```python
from build123d import *

# Parameters (mm, degrees)
F1_DEPTH = 40.64
F2_W     = 58.1915168336
F2_H     = 84.6826420166
F3_DEPTH = 100.584
F4_DEPTH = 25.4
F5_R     = 11.938
F6_DEPTH = 25.4
F7_R     = 11.938
F8_DEPTH = 25.4


# Not quite as in the source:
# - a feature names something its author has since deleted; it is built from what else it names


with BuildPart() as f1:
    # F0 (on Front) → F1 (new body)
    with BuildSketch(Plane.XZ):
        Polygon((5.0445693985, -63.1324924332), (45.3936140645, -28.3097998209), (45.3936140645, 92.1692103148), (-35.2877192199, 92.1692103148), (-35.2877192199, -28.3036921173), align=None)
    extrude(amount=F1_DEPTH)

    # F2 (on face) → F3 (cut)
    with BuildSketch(Plane.XZ.offset(40.64)):
        with Locations((5.3103963967, 34.6377051901)):
            Rectangle(F2_W, F2_H)
    extrude(amount=-F3_DEPTH, mode=Mode.SUBTRACT)

    # F2 (on face) → F4 (cut)
    with BuildSketch(Plane.XZ.offset(40.64)):
        with Locations((5.3103963967, 34.6377051901)):
            Rectangle(F2_W, F2_H)
    extrude(amount=-F4_DEPTH, mode=Mode.SUBTRACT)

    # F5 (on face) → F6 (cut)
    with BuildSketch(Plane(origin=(-35.2877192199, 0, 0), x_dir=(0, -1, 0), z_dir=(-1, 0, 0))):
        with Locations((19.3923822703, 31.1755515458)):
            Circle(F5_R)
    extrude(amount=-F6_DEPTH, mode=Mode.SUBTRACT)

    # F7 (on face) → F8 (cut)
    with BuildSketch(Plane.YZ.offset(45.3936140645)):
        with Locations((-19.7985949944, 31.1684036463)):
            Circle(F7_R)
    extrude(amount=-F8_DEPTH, mode=Mode.SUBTRACT)


solid = f1.part
```
Build history of the part. All positions in model axes, mm. A direction names the side the tool comes from. Give positions to 0.01 mm unless a question says otherwise; leave off trailing zeros. Order: outer loops, then holes, each group sorted by start corner. A loop starts at its lowest first (then second) coordinate and runs counter-clockwise, first axis right, second up. Notation, with made-up numbers: M -23.75,76.5 L -15.75,76.5 A19 ccw -15.75,95.5 Z; hole C 62,-35 d9. An arc over 180 degrees is marked long. Return JSON: item names as keys, results as strings.
Q1. Band-saw the part on C-C (x = 31.5). Give the cut face in (y, z), then the cut area to 3 significant figures.
Answer list:
{"outline": "M -40.64,-40.3 L 0,-40.3 L 0,-7.7 L -40.64,-7.7 Z; M -40.64,76.98 L 0,76.98 L 0,92.17 L -40.64,92.17 Z", "area": "1,940 mm^2"}
Q2. Band-saw the part on A-A (y = -4). Give the cut face in (x, z).
Answer list:
{"outline": "M -35.29,-28.3 L 5.04,-63.13 L 45.39,-28.31 L 45.39,92.17 L -35.29,92.17 Z; hole M -23.79,-7.7 L 34.41,-7.7 L 34.41,76.98 L -23.79,76.98 Z"}
Q3. 3-axis set-ups, long thin cutter, end or side, ignore diameter. For faces 5 (the face through (4, -40.64, -19)), 6 (the face through (39.977, -13.381, 41.235)), 7 (the face through (-29.62, -25.81, 41.24)), 8 (the face through (-23.785, -20.6, 43.5)), 9 (the face through (6, -20, 92.169)): which of +Z, -Z, +X, -X, +Y, -Y reach the whole face in a straight line?
Answer list:
{"face 5": "+Z, -Z, +X, -X, -Y", "face 6": "+X", "face 7": "-X", "face 8": "+Y, -Y", "face 9": "+Z, +X, -X, +Y, -Y"}
Q4. Wall check: probe 1 along X at (y, z) = (-35, 72.5); probe 2 along Z at (x, y) = (-21, -9.5); probe 3 along Z at (x, y) = (0, -14). Give the ranges that are in metal, low to high. Write a range as from..to.
Answer list:
{"probe 1": "x = -35.29..-23.79, 34.41..45.39", "probe 2": "z = -40.64..-7.7, 76.98..92.17", "probe 3": "z = -58.78..-7.7, 76.98..92.17"}
Q5. Band-saw the part on B-B (z = 47). Give the cut face in (x, y).
Answer list:
{"outline": "M -35.29,-40.64 L -23.79,-40.64 L -23.79,0 L -35.29,0 Z; M 34.41,-40.64 L 45.39,-40.64 L 45.39,0 L 34.41,0 Z"}
Q6. Band-saw the part on D-D (z = 29). Give the cut face in (x, y), then the cut area to 3 significant figures.
Answer list:
{"outline": "M -35.29,-40.64 L -23.79,-40.64 L -23.79,-31.13 L -35.29,-31.13 Z; M -35.29,-7.65 L -23.79,-7.65 L -23.79,0 L -35.29,0 Z; M 34.41,-40.64 L 45.39,-40.64 L 45.39,-31.54 L 34.41,-31.54 Z; M 34.41,-8.06 L 45.39,-8.06 L 45.39,0 L 34.41,0 Z", "area": "386 mm^2"}
Q7. Two-plate mould, pull along X, no slides. Class faces 1 (the face through (-35.288, -20, 46)), 2 (the face through (5, -21, 76.979)), 3 (the face through (5, -21, -7.704)), 4 (the face through (4, 0, -19)): pulls with the +X half, pulls with the -X half, needs draft (parallel to the pull), parting line crosses it, or undercut.
Answer list:
{"face 1": "pulls with the -X half", "face 2": "undercut", "face 3": "undercut", "face 4": "needs draft"}
Q8. Flat gauge pins, fed straight in: pin 1 (10 mm diameter, centred on y = -15.5, z = -45.5, fed in from -X); pin 2 (14.5 mm diameter, centred on y = -19.39, z = 31.18, fed in from +X); pin 3 (1 mm diameter, centred on x = 20, y = -34.5, fed in from -Z). Where does each tip first touch, or does it go through?
Answer list:
{"pin 1": "stops at x = -21.16", "pin 2": "passes through", "pin 3": "stops at z = -50.66"}
